from build123d import *

# Parameters (mm, degrees)
F0_R     = 10.16
F1_DEPTH = 15.7734
F2_R     = 28.575
F3_DEPTH = 40.2336
F4_SIZE  = 3.302


with BuildPart() as f1:
    # F0 (on Top) → F1 (new body)
    with BuildSketch(Plane.XY):
        with BuildLine():
            Line((57.336765, 18.751028), (5.042647, 28.126541))
            ThreePointArc((5.042647, 28.126541), (-28.575, 0), (5.042647, -28.126541))
            Line((5.042647, -28.126541), (57.336765, -18.751028))
            ThreePointArc((57.336765, -18.751028), (73.025, 0), (57.336765, 18.751028))
        make_face()
        with Locations((53.975, 0)):
            Circle(F0_R, mode=Mode.SUBTRACT)
    extrude(amount=F1_DEPTH)

    # F2 (on Top) → F3 (join)
    with BuildSketch(Plane.XY):
        Circle(F2_R)
        with BuildLine():
            ThreePointArc((13.447765, -4.826), (-14.2875, 0), (13.447765, 4.826))
            Line((13.447765, 4.826), (18.5293, 4.826))
            Line((18.5293, 4.826), (18.5293, -4.826))
            Line((18.5293, -4.826), (13.447765, -4.826))
        make_face(mode=Mode.SUBTRACT)
    extrude(amount=F3_DEPTH)

    # F4
    f4_edges = [f1.edges().sort_by_distance(p)[0] for p in [
        (-28.575, 0, 40.2336),
    ]]
    chamfer(f4_edges, length=F4_SIZE)


solid = f1.part
Model file for the job. Use its own axes, mm. A direction names the side the tool comes from. Coordinates: 2 decimals unless noted, no trailing zeros. Write each loop counter-clockwise with the first axis right and the second up, starting at its lowest first coordinate (ties: lowest second). Pieces come first, ordered by that corner, then holes. Notation, with made-up numbers: (19, 74) - (70, 74) arc R29 ccw to (70, 100) - close; hole circle Ø7 at (63.25, 62.5). An arc over 180 degrees is marked (long way). Write each question's results on one line, items separated by ' | '. Start each with the question number.
1) Mould opens along Y. For faces 1 (the face through (2, 0, 15.773)), 2 (the face through (16, 4.826, 28)), 3 (the face through (-28.547, 1.256, 22.311)), 4 (the face through (22, 0, 0)) say: pulls with the +Y half, pulls with the -Y half, needs draft (parallel to the pull), parting line crosses it, or undercut.
2) Flat gauge pins, fed straight in: P1, Ø4, axis at x = 34, y = -6.5, coming from the +Z side; P2, Ø1.5, axis at x = 16.5, z = 22.5, coming from the -Y side; P3, Ø4, axis at x = -6, z = 10, coming from the -Y side; P4, Ø23.5, axis at x = 53.975, y = 0, coming from the -Z side. Where does each tip first touch, or does it go through?
3) Cut at A-A (y = 0). Write the cut outline in (x, z) (1 decimal).
4) Cut at C-C (x = 54). Write the cut outline in (y, z).
5) 3-axis set-ups, long thin cutter, end or side, ignore diameter. For faces 5 (the face through (18.529, 0, 28)), 6 (the face through (31.558, 23.373, 7.776)): which of +Z, -Z, +X, -X, +Y, -Y reach the whole face in a straight line?
6) Cut at D-D (x = 0). Write the cut outline in (y, z) (1 decimal), then the cut area to 3 significant figures.
7) Probe line 1 along X through (y, z) = (0, 26.5) (1 decimal); line 2 along Y through (x, z) = (0, 29.75) (1 decimal); line 3 along Z through (x, y) = (-9.5, -4). List the from-to ranges inside material, lowest first. Write a range as from..to.
Returned:
1) face 1: undercut | face 2: undercut | face 3: parting line crosses it | face 4: needs draft
2) P1: z = 15.77 | P2: y = -23.84 | P3: y = -28.29 | P4: z = 0
3) outline: (-28.6, 0) - (43.8, 0) - (43.8, 15.8) - (28.6, 15.8) - (28.6, 36.9) - (25.3, 40.2) - (18.5, 40.2) - (18.5, 15.8) - (-14.3, 15.8) - (-14.3, 40.2) - (-25.3, 40.2) - (-28.6, 36.9) - close; (64.1, 0) - (73, 0) - (73, 15.8) - (64.1, 15.8) - close
4) outline: (-19.35, 0) - (-10.16, 0) - (-10.16, 15.77) - (-19.35, 15.77) - close; (10.16, 0) - (19.35, 0) - (19.35, 15.77) - (10.16, 15.77) - close
5) face 5: +Z | face 6: +Z, -Z, +X, +Y
6) outline: (-28.6, 0) - (28.6, 0) - (28.6, 36.9) - (25.3, 40.2) - (14.3, 40.2) - (14.3, 15.8) - (-14.3, 15.8) - (-14.3, 40.2) - (-25.3, 40.2) - (-28.6, 36.9) - close | area: 1,590 mm^2
7) line 1: -28.6..-14.3, 18.5..28.6 | line 2: -28.6..-14.3, 14.3..28.6 | line 3: 0..15.77
